```python
from build123d import *

# Parameters (mm, degrees)
SKETCH1_W                          = 170
SKETCH1_H                          = 97
BOSS_EXTRUDE1_DEPTH                = 10
FILLET1_R                          = 5
F_11_0_START                       = -10
F_11_0_11_DIAMETER_HOLE1_OUTLINE_R = 3
F_11_0_11_DIAMETER_HOLE1_DEPTH     = 10
SKETCH7_R                          = 5.5
CUT_EXTRUDE1_DEPTH                 = 4.5
M8_CLEARANCE_HOLE1_D               = 8.4
F_8_0MM_DOWEL_HOLE1_D              = 8


# Read off the part's stored shape, not the designer's step: Ø11.0 (11) Diameter Hole1
with BuildPart() as part:
    # Sketch1 → Boss-Extrude1 (new body)
    with BuildSketch(Plane(origin=(0, 0, 0), x_dir=(1, 0, 0), z_dir=(0, 1, 0))):
        Rectangle(SKETCH1_W, SKETCH1_H)
    extrude(amount=-BOSS_EXTRUDE1_DEPTH)

    # Fillet1
    fillet1_edges = [part.edges().sort_by_distance(p)[0] for p in [
        (85, -5, 48.5),
        (-85, -5, 48.5),
        (-85, -5, -48.5),
        (85, -5, -48.5),
    ]]
    fillet(fillet1_edges, radius=FILLET1_R)

    # Ø11.0 (11) Diameter Hole1 outline → Ø11.0 (11) Diameter Hole1 (cut)
    with BuildSketch(Plane(origin=(0, 0, 0), x_dir=(1, 0, 0), z_dir=(0, 1, 0)).offset(F_11_0_START)):
        with Locations((29, -22.5)):
            Circle(F_11_0_11_DIAMETER_HOLE1_OUTLINE_R)
        with Locations((-29, 22.5)):
            Circle(F_11_0_11_DIAMETER_HOLE1_OUTLINE_R)
        with Locations((-29, -22.5)):
            Circle(F_11_0_11_DIAMETER_HOLE1_OUTLINE_R)
        with Locations((29, 22.5)):
            Circle(F_11_0_11_DIAMETER_HOLE1_OUTLINE_R)
    extrude(amount=F_11_0_11_DIAMETER_HOLE1_DEPTH, mode=Mode.SUBTRACT)

    # Sketch7 → Cut-Extrude1 (cut)
    with BuildSketch(Plane(origin=(0, 0, 0), x_dir=(1, 0, 0), z_dir=(0, 1, 0))):
        with Locations(Location((-29, 22.5, 0), (0, 0, 270))):
            Circle(SKETCH7_R)
        with Locations(Location((29, 22.5, 0), (0, 0, 270))):
            Circle(SKETCH7_R)
        with Locations(Location((29, -22.5, 0), (0, 0, 270))):
            Circle(SKETCH7_R)
        with Locations(Location((-29, -22.5, 0), (0, 0, 270))):
            Circle(SKETCH7_R)
    extrude(amount=-CUT_EXTRUDE1_DEPTH, mode=Mode.SUBTRACT)

    # M8 Clearance Hole1 (through all)
    with Locations(Plane(origin=(0, 0, 0), x_dir=(1, 0, 0), z_dir=(0, 1, 0))):
        with Locations((-75, -38.5), (-75, 38.5), (75, -38.5), (75, 38.5)):
            Hole(M8_CLEARANCE_HOLE1_D / 2)

    # Ø8.0mm Dowel Hole1 (through all)
    with Locations(Plane(origin=(0, 0, 0), x_dir=(1, 0, 0), z_dir=(0, 1, 0))):
        with Locations((-75, 0), (75, 0)):
            Hole(F_8_0MM_DOWEL_HOLE1_D / 2)


solid = part.part
```
Could you check a few things on this model? Use its own coordinates, in mm. A direction names the side the tool comes from. Coordinates: 2 decimals unless noted, no trailing zeros. Write each loop counter-clockwise with the first axis right and the second up, starting at its lowest first coordinate (ties: lowest second). Pieces come first, ordered by that corner, then holes. Notation, with made-up numbers: (74.25, -11) - (103.25, -11) arc R15 cw to (103.25, 7) - close; hole circle Ø5 at (-3.5, 53). An arc over 180 degrees is marked (long way). Use a Markdown table: item, result.
Q1. I'm going to push flat-ended pins straight in: pin 1 Ø17.5 at (x, z) = (29, 22.5) entering from -Y; pin 2 Ø3.5 at (x, z) = (30.5, -20) entering from +Y; pin 3 Ø7.5 at (x, z) = (-75, 38.5) entering from +Y. Where does each tip first touch, or does it pass through?
Geometry check:
| item | result |
|---|---|
| pin 1 | stops at y = -10 |
| pin 2 | stops at y = -4.5 |
| pin 3 | passes through |
Q2. Imagine slicing it at C-C (y = -1.5). Count the separate pieces of the cut face and the enclosed holes in it, and give its area (3 significant figures).
Geometry check:
| item | result |
|---|---|
| separate pieces | 1 |
| enclosed holes | 10 |
| area | 15,800 mm2 |
Q3. Which directions (+Z, -Z, +X, -X, +Y, -Y) give clear straight access to the entire face, cutting with the end or side of a thin tool? Please do faces 1 (the flat face through (27, -4.5, 25)), 2 (the flat face through (-1, -5, -48.5)).
Geometry check:
| item | result |
|---|---|
| face 1 | +Y |
| face 2 | -Z, +X, -X, +Y, -Y |
Q4. Please list where these lines run through material, in increasing order: L1, parallel to Z at x = 75, y = -6.75; L2, parallel to Z at x = -29, y = -8; L3, parallel to X at y = -8, z = 22.5.
Geometry check:
| item | result |
|---|---|
| L1 | z = -48.5 to -42.7, -34.3 to -4, 4 to 34.3, 42.7 to 48.5 |
| L2 | z = -48.5 to -25.5, -19.5 to 19.5, 25.5 to 48.5 |
| L3 | x = -85 to -32, -26 to 26, 32 to 85 |
Q5. Imagine slicing it at B-B (z = -22.5). List the corners of the cut face in (x, y) for me, and give its area (4 significant figures).
Geometry check:
| item | result |
|---|---|
| outline | (-85, -10) - (-32, -10) - (-32, -4.5) - (-34.5, -4.5) - (-34.5, 0) - (-85, 0) - close; (-26, -10) - (26, -10) - (26, -4.5) - (23.5, -4.5) - (23.5, 0) - (-23.5, 0) - (-23.5, -4.5) - (-26, -4.5) - close; (32, -10) - (85, -10) - (85, 0) - (34.5, 0) - (34.5, -4.5) - (32, -4.5) - close |
| area | 1,535 mm2 |
Q6. Imagine slicing it at A-A (x = -75). List the corners of the cut face in (y, z) for me.
Geometry check:
| item | result |
|---|---|
| outline | (-10, -48.5) - (0, -48.5) - (0, -42.7) - (-10, -42.7) - close; (-10, -34.3) - (0, -34.3) - (0, -4) - (-10, -4) - close; (-10, 4) - (0, 4) - (0, 34.3) - (-10, 34.3) - close; (-10, 42.7) - (0, 42.7) - (0, 48.5) - (-10, 48.5) - close |
Q7. Imagine slicing it at D-D (x = 29). List the corners of the cut face in (y, z) for me.
Geometry check:
| item | result |
|---|---|
| outline | (-10, -48.5) - (0, -48.5) - (0, -28) - (-4.5, -28) - (-4.5, -25.5) - (-10, -25.5) - close; (-10, -19.5) - (-4.5, -19.5) - (-4.5, -17) - (0, -17) - (0, 17) - (-4.5, 17) - (-4.5, 19.5) - (-10, 19.5) - close; (-10, 25.5) - (-4.5, 25.5) - (-4.5, 28) - (0, 28) - (0, 48.5) - (-10, 48.5) - close |
Q8. Thinking about a two-plate mould opening in X: for faces 3 (the flat face through (-85, -5, 1)), 4 (the flat face through (-1, -10, -1)), 5 (the cylindrical face through (34.453, -2.218, 21.784)), 6 (the cylindrical face through (83.5, -5.07, 47.07)), which applies, +X half, -X half, draft (parallel to the pull), parting line (faces both ways), or undercut?
Geometry check:
| item | result |
|---|---|
| face 3 | -X half |
| face 4 | draft |
| face 5 | undercut |
| face 6 | +X half |
